Geometry: see drawing. Coordinates: mm, zero at the bounding-box minimum. Give positions to 0.01 mm unless a question says otherwise; leave off trailing zeros. Write each loop counter-clockwise with the first axis right and the second up, starting at its lowest first coordinate (ties: lowest second). Pieces come first, ordered by that corner, then holes. Notation, with made-up numbers: (-33, 48) -> (16, 48) arc R35 cw to (16, 82) -> close; hole circle Ø10 at (26.25, 32.5). An arc over 180 degrees is marked (long way). Answer as a JSON object with one key per item and string values. Group by question number.
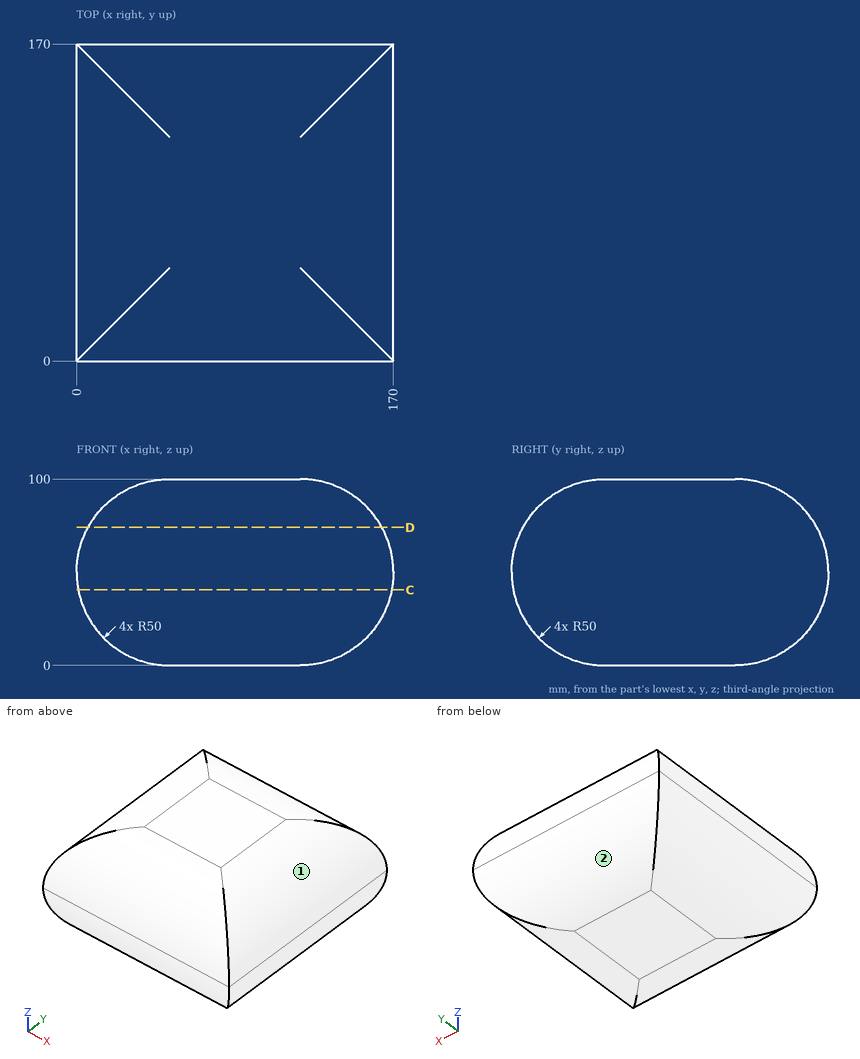
1. Mould query, pull axis Z, two halves, no side actions, for the marked faces 1 and 2. Classes: pulls with the +Z half, pulls with the -Z half, needs draft (parallel to the pull), parting line crosses it, or undercut.
2. Contact query for flat-ended pins moving along their axis: pin 1 Ø8 at (y, z) = (73.5, 56) entering from +X; pin 2 Ø5 at (x, z) = (139, 27.5) entering from +Y; pin 3 Ø10 at (y, z) = (25.5, 19.5) entering from +X. Output: stop coordinate, or through.
3. Section C-C (z = 40.5). Return the cut outline in (x, y), plus the area to 3 significant figures.
4. Line query: line 1 (Y direction, x = 51, z = 14); line 2 (Z direction, x = 152, y = 15); line 3 (Z direction, x = 38, y = 105). Output: solid intervals per line, ascending.
5. Section D-D (z = 74). Return the cut outline in (x, y).
Working result:
{
 "1": {"face 1": "pulls with the +Z half", "face 2": "pulls with the -Z half"},
 "2": {"pin 1": "stops at x = 169.96", "pin 2": "stops at y = 165.83", "pin 3": "stops at x = 163.01"},
 "3": {"outline": "(0.91, 0.91) -> (169.09, 0.91) -> (169.09, 169.09) -> (0.91, 169.09) -> close", "area": "28,300 mm^2"},
 "4": {"line 1": "y = 15.3 to 154.7", "line 2": "z = 14.29 to 85.71", "line 3": "z = 1.46 to 98.54"},
 "5": {"outline": "(6.14, 6.14) -> (163.86, 6.14) -> (163.86, 163.86) -> (6.14, 163.86) -> close"}
}
